```python
from build123d import *

# Parameters (mm, degrees)
SKETCH_1_W                       = 8
SKETCH_1_H                       = 8
HEIGHT_DEPTH                     = 3.2
SKETCH_2_R                       = 2.4
EXTRUDE_2_DEPTH                  = 1.7
PATTERN_LINEAR_1_COUNT           = 2
PATTERN_LINEAR_1_PITCH           = 8
PATTERN_LINEAR_2_COUNT           = 4
PATTERN_LINEAR_2_PITCH           = 8
PATTERN_LINEAR_2_COPY_1_SKETCH_W = 8
PATTERN_LINEAR_2_COPY_1_SKETCH_H = 8
PATTERN_LINEAR_2_COPY_1_DEPTH    = 3.2
PATTERN_LINEAR_2_COPY_2_SKETCH_W = 8
PATTERN_LINEAR_2_COPY_2_SKETCH_H = 8
PATTERN_LINEAR_2_COPY_2_DEPTH    = 3.2
PATTERN_LINEAR_2_COPY_3_SKETCH_W = 8
PATTERN_LINEAR_2_COPY_3_SKETCH_H = 8
PATTERN_LINEAR_2_COPY_3_DEPTH    = 3.2
PATTERN_LINEAR_2_COPY_4_SKETCH_R = 2.4
PATTERN_LINEAR_2_COPY_4_DEPTH    = 1.7
PATTERN_LINEAR_2_COPY_5_SKETCH_R = 2.4
PATTERN_LINEAR_2_COPY_5_DEPTH    = 1.7
PATTERN_LINEAR_2_COPY_6_SKETCH_R = 2.4
PATTERN_LINEAR_2_COPY_6_DEPTH    = 1.7
SHELL_1_T                        = -1.6
SKETCH_3_R                       = 3.255
SKETCH_3_R_2                     = 2.4
EXTRUDE_3_DEPTH                  = 1.6
PATTERN_LINEAR_3_COUNT           = 3
PATTERN_LINEAR_3_PITCH           = 8


with BuildPart() as part:
    # 草圖1 → height (new body)
    with BuildSketch(Plane(origin=(0, 0, 0), x_dir=(1, 0, 0), z_dir=(0, 1, 0))):
        Rectangle(SKETCH_1_W, SKETCH_1_H)
    height = extrude(amount=HEIGHT_DEPTH)

    # 草圖2 → 填料-伸長2 (add)
    with BuildSketch(Plane(origin=(0, 3.2, 0), x_dir=(1, 0, 0), z_dir=(0, 1, 0))):
        Circle(SKETCH_2_R)
    extrude_2 = extrude(amount=EXTRUDE_2_DEPTH)

    # 直線複製排列1: height, 填料-伸長2 ×2
    with Locations(*[(0, 0, i * PATTERN_LINEAR_1_PITCH) for i in range(1, PATTERN_LINEAR_1_COUNT)]):
        add(height)
        add(extrude_2)

    # 直線複製排列2: height, 填料-伸長2 ×4
    with Locations(*[(i * PATTERN_LINEAR_2_PITCH, 0, 0) for i in range(1, PATTERN_LINEAR_2_COUNT)]):
        add(height)
        add(extrude_2)

    # 直線複製排列2 copy 1 sketch → 直線複製排列2 copy 1 (add)
    with BuildSketch(Plane(origin=(8, 0, 8), x_dir=(1, 0, 0), z_dir=(0, 1, 0))):
        Rectangle(PATTERN_LINEAR_2_COPY_1_SKETCH_W, PATTERN_LINEAR_2_COPY_1_SKETCH_H)
    extrude(amount=PATTERN_LINEAR_2_COPY_1_DEPTH)

    # 直線複製排列2 copy 2 sketch → 直線複製排列2 copy 2 (add)
    with BuildSketch(Plane(origin=(16, 0, 8), x_dir=(1, 0, 0), z_dir=(0, 1, 0))):
        Rectangle(PATTERN_LINEAR_2_COPY_2_SKETCH_W, PATTERN_LINEAR_2_COPY_2_SKETCH_H)
    extrude(amount=PATTERN_LINEAR_2_COPY_2_DEPTH)

    # 直線複製排列2 copy 3 sketch → 直線複製排列2 copy 3 (add)
    with BuildSketch(Plane(origin=(24, 0, 8), x_dir=(1, 0, 0), z_dir=(0, 1, 0))):
        Rectangle(PATTERN_LINEAR_2_COPY_3_SKETCH_W, PATTERN_LINEAR_2_COPY_3_SKETCH_H)
    extrude(amount=PATTERN_LINEAR_2_COPY_3_DEPTH)

    # 直線複製排列2 copy 4 sketch → 直線複製排列2 copy 4 (add)
    with BuildSketch(Plane(origin=(8, 3.2, 8), x_dir=(1, 0, 0), z_dir=(0, 1, 0))):
        Circle(PATTERN_LINEAR_2_COPY_4_SKETCH_R)
    extrude(amount=PATTERN_LINEAR_2_COPY_4_DEPTH)

    # 直線複製排列2 copy 5 sketch → 直線複製排列2 copy 5 (add)
    with BuildSketch(Plane(origin=(16, 3.2, 8), x_dir=(1, 0, 0), z_dir=(0, 1, 0))):
        Circle(PATTERN_LINEAR_2_COPY_5_SKETCH_R)
    extrude(amount=PATTERN_LINEAR_2_COPY_5_DEPTH)

    # 直線複製排列2 copy 6 sketch → 直線複製排列2 copy 6 (add)
    with BuildSketch(Plane(origin=(24, 3.2, 8), x_dir=(1, 0, 0), z_dir=(0, 1, 0))):
        Circle(PATTERN_LINEAR_2_COPY_6_SKETCH_R)
    extrude(amount=PATTERN_LINEAR_2_COPY_6_DEPTH)

    # 薄殼1
    shell_1_openings = [part.faces().sort_by_distance(p)[0] for p in [
        (12, 0, 4),
    ]]
    offset(amount=SHELL_1_T, openings=shell_1_openings, kind=Kind.INTERSECTION)

    # 草圖3 → 填料-伸長3 (add)
    with BuildSketch(Plane.XZ.offset(-1.6)):
        with Locations((4, 4)):
            Circle(SKETCH_3_R)
        with Locations((4, 4)):
            Circle(SKETCH_3_R_2, mode=Mode.SUBTRACT)
    extrude_3 = extrude(amount=EXTRUDE_3_DEPTH)

    # 直線複製排列3: 填料-伸長3 ×3
    with Locations(*[(i * PATTERN_LINEAR_3_PITCH, 0, 0) for i in range(1, PATTERN_LINEAR_3_COUNT)]):
        add(extrude_3)


solid = part.part
```
Geometry check sheet. Reference: the model listing, model coordinates, mm. A direction names the side the tool comes from. Coordinates: 2 decimals unless noted, no trailing zeros. Loops run counter-clockwise (first coordinate to the right, second up) from the corner with the lowest first, then second, coordinate; pieces in that order, holes last. Notation, with made-up numbers: (19.5, 63.25) - (28.5, 63.25) arc R15 ccw to (28.5, 92.25) - close; hole circle Ø10 at (14, 62). An arc over 180 degrees is marked (long way). One line per item, written item: value. Start each with the question number.
(1) Cross-section at A-A on y = 0.9. Enter the section's corners in (x, z) (3 decimals), plus the area to 3 significant figures.
(2) Cross-section at C-C on x = 8. Enter the section's corners in (y, z).
(3) Tool access check on faces 1 (the cylindrical face through (1.29, 4.038, 5.976)), 2 (the cylindrical face through (17.602, 0.811, 4.106)), 3 (the flat face through (28, 2, 4)). Record the directions out of +Z, -Z, +X, -X, +Y, -Y that give a thin tool (end or side, any length) a straight path to the whole face; none if there is none.
(4) Cross-section at B-B on y = 2.45. Count the separate pieces of the cut face and the enclosed holes in it, plus the area to 3 significant figures.
(5) Cross-section at D-D on z = -2. Enter the section's corners in (x, y), plus the area to 3 significant figures.
(6) Material ranges on line 1 (Z direction, x = 0, y = 2.45); line 2 (Z direction, x = 0, y = 4.55); line 3 (Z direction, x = 20, y = 0.6) (3 decimals), recorded low to high. Write a range as [from, to].
(7) Mould release check, pull along Z, two halves, no side actions. Record for faces 4 (the flat face through (8, 4.9, 8)), 5 (the cylindrical face through (7.41, 2.44, 7.46)): released by +Z, released by -Z, zero draft, split by the parting line, or undercut.
(8) Depth check by flat-ended pin: P1, Ø1.3, axis at x = 16.5, z = 0, coming from the -Y side; P2, Ø1.3, axis at x = 8, z = 8, coming from the -Y side. Enter the tip coordinate at first touch or a pass-through.
Results below:
1. outline: (-4, -4) - (28, -4) - (28, 12) - (-4, 12) - close; circle Ø6.51 at (4, 4); circle Ø6.51 at (12, 4); circle Ø6.51 at (20, 4); hole (-2.4, -2.4) - (26.4, -2.4) - (26.4, 10.4) - (-2.4, 10.4) - close; hole circle Ø4.8 at (4, 4); hole circle Ø4.8 at (12, 4); hole circle Ø4.8 at (20, 4)
1. area: 189 mm2
2. outline: (0, -4) - (3.2, -4) - (3.2, -2.4) - (4.9, -2.4) - (4.9, 2.4) - (3.2, 2.4) - (3.2, 5.6) - (4.9, 5.6) - (4.9, 10.4) - (3.2, 10.4) - (3.2, 12) - (0, 12) - (0, 10.4) - (1.6, 10.4) - (1.6, 8.8) - (3.3, 8.8) - (3.3, 7.2) - (1.6, 7.2) - (1.6, 0.8) - (3.3, 0.8) - (3.3, -0.8) - (1.6, -0.8) - (1.6, -2.4) - (0, -2.4) - close
3. face 1: +Y
3. face 2: -Y
3. face 3: +Z, -Z, +X, +Y, -Y
4. separate pieces: 1
4. enclosed holes: 8
4. area: 496 mm2
5. outline: (-4, 0) - (-2.4, 0) - (-2.4, 1.6) - (26.4, 1.6) - (26.4, 0) - (28, 0) - (28, 3.2) - (25.33, 3.2) - (25.33, 4.9) - (22.67, 4.9) - (22.67, 3.2) - (17.33, 3.2) - (17.33, 4.9) - (14.67, 4.9) - (14.67, 3.2) - (9.33, 3.2) - (9.33, 4.9) - (6.67, 4.9) - (6.67, 3.2) - (1.33, 3.2) - (1.33, 4.9) - (-1.33, 4.9) - (-1.33, 3.2) - (-4, 3.2) - close
5. area: 74.4 mm2
6. line 1: z = [-4, -0.8], [0.8, 7.2], [8.8, 12]
6. line 2: z = [-2.4, 2.4], [5.6, 10.4]
6. line 3: z = [-4, -2.4], [0.745, 1.6], [6.4, 7.255], [10.4, 12]
7. face 4: zero draft
7. face 5: undercut
8. P1: stops at y = 1.6
8. P2: stops at y = 3.3
